Drawing for the job (mm, zero at the part's lowest x, y, z). A direction names the side the tool comes from. Coordinates: 2 decimals unless noted, no trailing zeros. Loops run counter-clockwise (first coordinate to the right, second up) from the corner with the lowest first, then second, coordinate; pieces in that order, holes last. Notation, with made-up numbers: (79, -40) - (96, -40) arc R23 cw to (96, -8) - close; hole circle Ø9 at (20.5, 55.25). An arc over 180 degrees is marked (long way). Put each result on its own line as item: value.
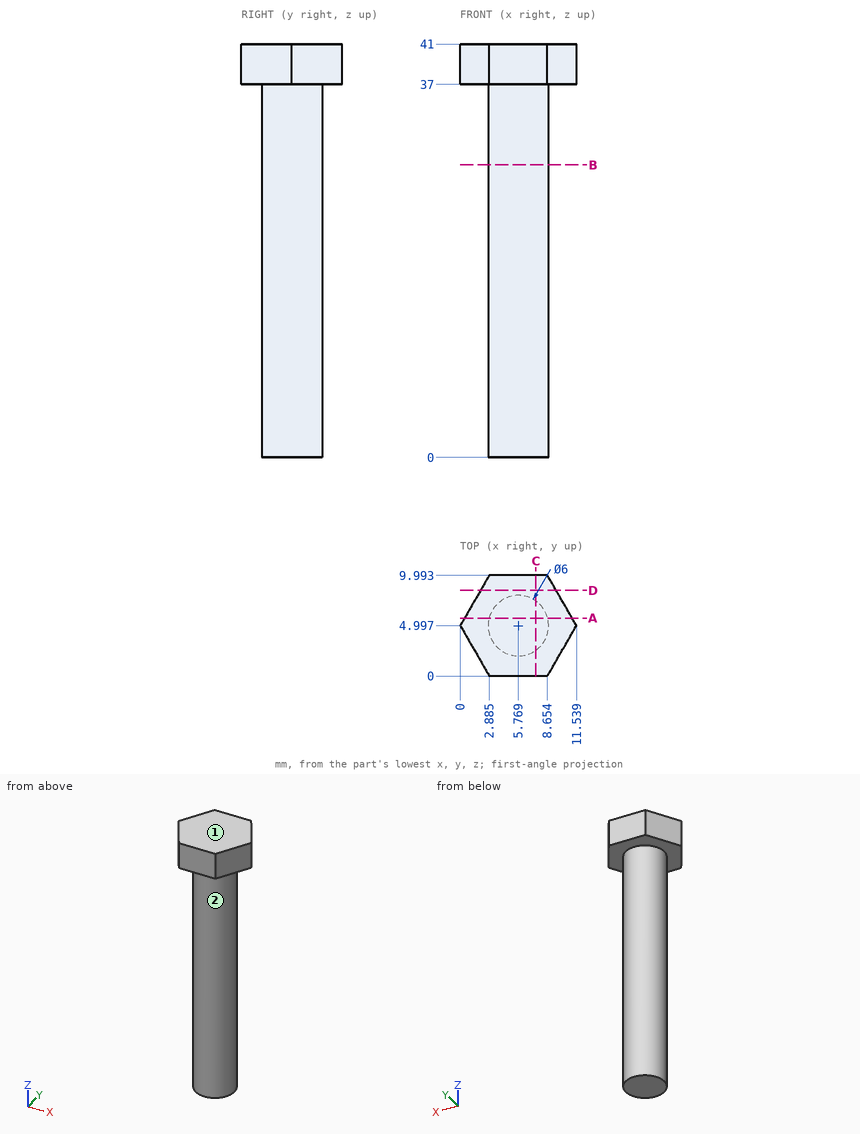
Q1. Slice it at B-B, the plane z = 29. Give the cut face in (x, y), then the cut area to 3 significant figures.
Determined:
outline: circle Ø6 at (5.77, 5)
area: 28.3 mm2
Q2. Tool access for the marked faces 1 and 2: list every direction of +Z, -Z, +X, -X, +Y, -Y with a clear straight run to the whole face (end or side of a thin tool).
Determined:
face 1: +Z, +X, -X, +Y, -Y
face 2: -Z
Q3. Pin check, flat tips, straight feed: pin 1 Ø4 at (y, z) = (1.5, 29) entering from +X; pin 2 Ø5 at (x, z) = (6.5, 29.5) entering from +Y; pin 3 Ø3 at (y, z) = (6.5, 25) entering from +X. Stop position of each tip, or through.
Determined:
pin 1: x = 8.37
pin 2: y = 8
pin 3: x = 8.77
Q4. Slice it at C-C, the plane x = 7.5. Give the cut face in (y, z) (1 decimal).
Determined:
outline: (0, 37) - (2.5, 37) - (2.5, 0) - (7.4, 0) - (7.4, 37) - (10, 37) - (10, 41) - (0, 41) - close
Q5. Slice it at A-A, the plane y = 5.75. Give the cut face in (x, z) (1 decimal).
Determined:
outline: (0.4, 37) - (2.9, 37) - (2.9, 0) - (8.7, 0) - (8.7, 37) - (11.1, 37) - (11.1, 41) - (0.4, 41) - close
Q6. Slice it at D-D, the plane y = 8.5. Give the cut face in (x, z), then the cut area to 3 significant figures.
Determined:
outline: (2.02, 37) - (9.52, 37) - (9.52, 41) - (2.02, 41) - close
area: 30.0 mm2
Q7. Wall check: L1, parallel to Z at x = 5.75, y = 9; L2, parallel to Y at x = 3.75, z = 20 (1 decimal); L3, parallel to X at y = 7.75, z = 38. Give the ranges that are in metal, low to high. Write a range as from..to.
Determined:
L1: 37..41
L2: 2.8..7.2
L3: 1.59..9.95
